Autodesk Inventor part; units mm, degrees
ref_plane "YZ Plane" through (0, 0, 0) normal (1, 0, 0) x (0, 1, 0)
ref_plane "XZ Plane" through (0, 0, 0) normal (0, 1, 0) x (-1, 0, 0)
ref_plane "XY Plane" through (0, 0, 0) normal (0, 0, 1) x (1, 0, 0)
sketch "Sketch1" plane through (0, 0, 0) normal (0, 0, 1) x (1, 0, 0)
  line L0 (0, 0) -> (254, 0)
  line L1 (0, 50.8) -> (254, 50.8)
  arc A0 (0, 50.8) -> (0, 0) centre (0, 25.4) ccw
  line L2 (254, 50.8) -> (290.3943, 25.4)
  line L3 (290.3943, 25.4) -> (254, 0)
  circle A1 centre (0, 25.4) radius 12.7
  dimension "d0" = 254
  dimension "d1" = 254
  dimension "d2" = 50.8
  dimension "d3" = 25.4
  dimension "d4" = 25.4
extrude "Extrusion1" add sketch "Sketch1" along normal blind 25.4 contours A0 L1 L2 L3 L0 | A1
sketch "Sketch2" plane through (0, 0, 25.4) normal (0, 0, 1) x (1, 0, 0)
  circle A0 centre (0, 25.4) radius 12.7
  arc A1 (0, 50.8) -> (0, 0) centre (0, 25.4) ccw
  dimension "d7" = 25.4
extrude "Extrusion2" add sketch "Sketch2" along normal blind 25.4
properties part number "Punta de flecha"
Geometry: final body of the model. Coordinates: model frame, mm. A direction names the side the tool comes from. Give positions to 0.01 mm unless a question says otherwise; leave off trailing zeros. Write each loop counter-clockwise with the first axis right and the second up, starting at its lowest first coordinate (ties: lowest second). Pieces come first, ordered by that corner, then holes. Notation, with made-up numbers: (29, 86) -> (85, 86) arc R11 cw to (85, 100) -> close; hole circle Ø1 at (86, 54). An arc over 180 degrees is marked (long way). Answer in a Markdown table with one row per item.
(1) Section query B-B on y = 30. Return loops of the section in (x, z).
Answers below:
| item | result |
|---|---|
| outline | (-24.98, 0) -> (283.8, 0) -> (283.8, 25.4) -> (11.84, 25.4) -> (11.84, 50.8) -> (-11.84, 50.8) -> (-11.84, 25.4) -> (-24.98, 25.4) -> close |
(2) Ray query, line 1 along X through (y, z) = (26.5, 45.5); line 2 along Z through (x, y) = (68, 18); line 3 along X through (y, z) = (28, 40). Return the intervals inside material, ascending. Write a range as [from, to].
Answers below:
| item | result |
|---|---|
| line 1 | [-12.65, 12.65] |
| line 2 | [0, 25.4] |
| line 3 | [-12.43, 12.43] |
(3) Set-up query: faces 1 (the flat face through (125, 50.8, 13)), 2 (the cylindrical face through (-2.75, 37.8, 37.92)). Return all of +Z, -Z, +X, -X, +Y, -Y with unobstructed straight access to the full face (end or side cutting, diameter ignored); none if empty.
Answers below:
| item | result |
|---|---|
| face 1 | +Z, -Z, +X, -X, +Y |
| face 2 | +Z |
(4) Section query C-C on x = 162.5. Return loops of the section in (y, z), then the cut area to 3 significant figures.
Answers below:
| item | result |
|---|---|
| outline | (0, 0) -> (50.8, 0) -> (50.8, 25.4) -> (0, 25.4) -> close |
| area | 1,290 mm^2 |
(5) Section query A-A on z = 15. Return loops of the section in (x, y).
Answers below:
| item | result |
|---|---|
| outline | (0, 0) -> (254, 0) -> (290.39, 25.4) -> (254, 50.8) -> (0, 50.8) arc R25.4 ccw to start |
(6) Section query D-D on z = 42. Return loops of the section in (x, y).
Answers below:
| item | result |
|---|---|
| outline | circle Ø25.4 at (0, 25.4) |
(7) Pin query (flat end, axial travel): pin 1 (8 mm diameter, centred on y = 42.5, z = 21.5, fed in from +X); pin 2 (2 mm diameter, centred on y = 12, z = 23.5, fed in from -X); pin 3 (15 mm diameter, centred on x = 78, y = 34, fed in from +Z). Return the tip coordinate at first contact, or that it passes through.
Answers below:
| item | result |
|---|---|
| pin 1 | x = 271.62 |
| pin 2 | x = -22.17 |
| pin 3 | z = 25.4 |
